from build123d import *

# Parameters (mm, degrees)
BOSS_EXTRUDE1_DEPTH = 25
SKETCH2_R           = 2.5
CUT_EXTRUDE1_DEPTH  = 4
SKETCH5_R           = 5
CUT_EXTRUDE2_DEPTH  = 60
SKETCH5_3_R         = 5
CUT_EXTRUDE3_DEPTH  = 5


with BuildPart() as part:
    # Sketch1 → Boss-Extrude1 (new body, symmetric)
    with BuildSketch(Plane(origin=(0, 0, 0), x_dir=(0, 0, -1), z_dir=(1, 0, 0))):
        with BuildLine():
            Line((0, 27), (0, -27))
            ThreePointArc((0, -27), (-0.878679656, -29.121320344), (-3, -30))
            Line((-3, -30), (-24, -30))
            Line((-24, -30), (-24, -25))
            Line((-24, -25), (-7, -25))
            ThreePointArc((-7, -25), (-4.878679656, -24.121320344), (-4, -22))
            Line((-4, -22), (-4, 22))
            ThreePointArc((-4, 22), (-4.878679656, 24.121320344), (-7, 25))
            Line((-7, 25), (-24, 25))
            Line((-24, 25), (-24, 30))
            Line((-24, 30), (-3, 30))
            ThreePointArc((-3, 30), (-0.878679656, 29.121320344), (0, 27))
        make_face()
    extrude(amount=BOSS_EXTRUDE1_DEPTH, both=True)

    # Sketch2 → Cut-Extrude1 (cut)
    with BuildSketch(Plane(origin=(0, 0, 0), x_dir=(-1, 0, 0), z_dir=(0, 0, -1))):
        Circle(SKETCH2_R)
        with Locations((0, 15)):
            Circle(SKETCH2_R)
        with Locations((10.606601718, 10.606601718)):
            Circle(SKETCH2_R)
        with Locations((-10.606601718, -10.606601718)):
            Circle(SKETCH2_R)
        with Locations((0, -15)):
            Circle(SKETCH2_R)
    extrude(amount=-CUT_EXTRUDE1_DEPTH, mode=Mode.SUBTRACT)

    # Sketch5 → Cut-Extrude2 (cut)
    with BuildSketch(Plane.XZ.offset(30)):
        with Locations((-15, 14)):
            Circle(SKETCH5_R)
    extrude(amount=-CUT_EXTRUDE2_DEPTH, mode=Mode.SUBTRACT)

    # Sketch5<3> → Cut-Extrude3 (cut)
    with BuildSketch(Plane.XZ.offset(30)):
        with Locations((15, 14)):
            Circle(SKETCH5_3_R)
    extrude(amount=-CUT_EXTRUDE3_DEPTH, mode=Mode.SUBTRACT)


solid = part.part
Geometry: final body of the model. Coordinates: model frame, mm. A direction names the side the tool comes from. Round coordinates to 2 decimals unless told otherwise and drop trailing zeros. Loops run counter-clockwise (first coordinate to the right, second up) from the corner with the lowest first, then second, coordinate; pieces in that order, holes last.
Q1. Section A-A on x = 0. Return loops of the section in (y, z).
Q2. Material intervals for L1, parallel to Y at x = 0, z = 2.85; L2, parallel to Y at x = 0, z = 2.35; L3, parallel to Y at x = 9, z = 20.5, sorted ascending.
Q3. Section C-C on x = 18. Return loops of the section in (y, z).
Q4. Access query for faces 5 (the cylindrical face through (0.35, 24.1, 4.86)), 6 (the cylindrical face through (19.619, -27.535, 12.085)), 7 (the flat face through (25, 0.4, 3.8)). Directions: +Z, -Z, +X, -X, +Y, -Y. A direction counts if a zero-diameter tool reaches every point of the face in a straight line with its end or side. Return the directions, or none.
Q5. Pin query (flat end, axial travel): P1, Ø8, axis at x = -7.5, y = 1, coming from the +Z side; P2, Ø9, axis at x = 15, z = 14, coming from the -Y side. Return the tip coordinate at first contact, or that it passes through.
Q6. Section D-D on z = 14. Return loops of the section in (x, y), plus the area to 3 significant figures.
Q7. Section B-B on y = 0. Return loops of the section in (x, z), plus the area to 3 significant figures.
Q8. Pull-direction query (Y, two-part tool) for faces 1 (the flat face through (0, -28, 24)), 2 (the cylindrical face through (0.54, -17.44, 1.97)), 3 (the cylindrical face through (0.35, -29.1, 0.86)), 4 (the cylindrical face through (12.45, -8.92, 1.97)); classes: released by +Y, released by -Y, zero draft, split by the parting line, or undercut.
Evaluation:
1. outline: (-30, 3) arc R3 ccw to (-27, 0) - (-17.5, 0) - (-17.5, 4) - (-22, 4) arc R3 cw to (-25, 7) - (-25, 24) - (-30, 24) - close; (-12.5, 0) - (-2.5, 0) - (-2.5, 4) - (-12.5, 4) - close; (2.5, 0) - (12.5, 0) - (12.5, 4) - (2.5, 4) - close; (17.5, 0) - (27, 0) arc R3 ccw to (30, 3) - (30, 24) - (25, 24) - (25, 7) arc R3 cw to (22, 4) - (17.5, 4) - close
2. L1: y = -30 to -17.5, -12.5 to -2.5, 2.5 to 12.5, 17.5 to 30
2. L2: y = -29.93 to -17.5, -12.5 to -2.5, 2.5 to 12.5, 17.5 to 29.93
2. L3: y = -30 to -25, 25 to 30
3. outline: (-30, 3) arc R3 ccw to (-27, 0) - (27, 0) arc R3 ccw to (30, 3) - (30, 24) - (25, 24) - (25, 7) arc R3 cw to (22, 4) - (-22, 4) arc R3 cw to (-25, 7) - (-25, 10) - (-30, 10) - close; (-30, 18) - (-25, 18) - (-25, 24) - (-30, 24) - close
4. face 5: +Z, +X, -X
4. face 6: -Y
4. face 7: +Z, -Z, +X, +Y, -Y
5. P1: stops at z = 4
5. P2: stops at y = 25
6. outline: (-25, -30) - (-20, -30) - (-20, -25) - (-25, -25) - close; (-25, 25) - (-20, 25) - (-20, 30) - (-25, 30) - close; (-10, -30) - (10, -30) - (10, -25) - (-10, -25) - close; (-10, 25) - (25, 25) - (25, 30) - (-10, 30) - close; (20, -30) - (25, -30) - (25, -25) - (20, -25) - close
6. area: 350 mm2
7. outline: (-25, 0) - (-2.5, 0) - (-2.5, 4) - (-25, 4) - close; (2.5, 0) - (25, 0) - (25, 4) - (2.5, 4) - close
7. area: 180 mm2
8. face 1: zero draft
8. face 2: undercut
8. face 3: released by -Y
8. face 4: undercut
